For this review, take the finished solid that the model builds, in its own axes (mm). Face numbers are marked on the shaded views. A direction names the side the tool comes from. Round coordinates to 2 decimals unless told otherwise and drop trailing zeros. Loops run counter-clockwise (first coordinate to the right, second up) from the corner with the lowest first, then second, coordinate; pieces in that order, holes last.
1) Tool access review of the marked faces 4 and 5: name each direction out of +Z, -Z, +X, -X, +Y, -Y from which nothing blocks a thin tool from reaching the whole face with its end or side.
2) Take a section at B-B (x = 44.5). State the section outline as (y, z) points, then the cut area to 3 significant figures.
3) Insertion check: pin 1 (10 mm diameter, centred on y = -3, z = -6.5, fed in from -X); pin 2 (7.5 mm diameter, centred on x = 145, y = 5, fed in from +Z); pin 3 (6 mm diameter, centred on y = -7, z = -2.5, fed in from +X); pin 4 (5 mm diameter, centred on x = 139, y = 2, fed in from -Z). Each pin has a flat end and moves straight along its axis. Give the tip position at first contact, or say it passes through.
4) Mouldability with a two-part tool opening along X and no side actions: class the marked faces 1, 2 and 3 as pulls with the +X half, pulls with the -X half, needs draft (parallel to the pull), parting line crosses it, or undercut.
5) Take a section at A-A (x = 16). State the section outline as (y, z) points, then the cut area to 3 significant figures.
6) Wall thickness on L1, parallel to Z at x = 111, y = -9; L2, parallel to Y at x = 147, z = 1.5; L3, parallel to Z at x = 70.5, y = -5.75: over which ranges is each line inside the solid? List them lowest first.
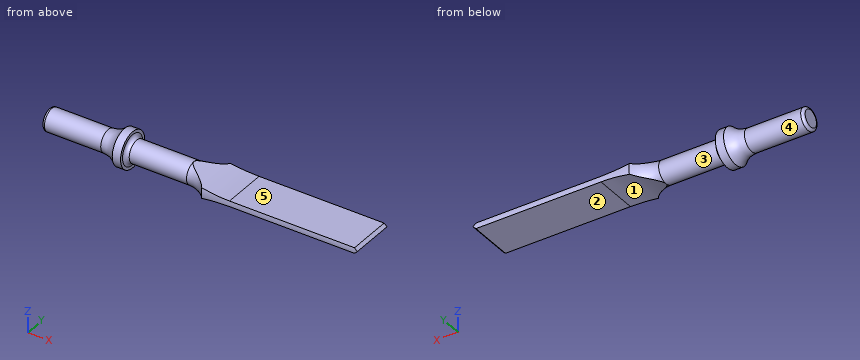
```python
from build123d import *

# Parameters (mm, degrees)
F3_DEPTH = 25.4
F4_DEPTH = 25.4
F6_DEPTH = 25.4
F7_DEPTH = 25.4


with BuildPart() as f1:
    # F0 (on Front) → F1 (revolve)
    with BuildSketch(Plane.XZ):
        with BuildLine():
            Line((0, 4.826), (0, 0))
            Line((0, 0), (184.15, 0))
            Line((184.15, 0), (184.15, 12.7))
            Line((184.15, 12.7), (95.25, 12.7))
            ThreePointArc((95.25, 12.7), (89.649516, 8.025968), (82.55, 6.35))
            Line((82.55, 6.35), (49.8856, 6.35))
            ThreePointArc((49.8856, 6.35), (48.269154, 7.019554), (47.5996, 8.636))
            Line((47.5996, 8.636), (47.5996, 10.3124))
            Line((47.5996, 10.3124), (42.8498, 10.3124))
            ThreePointArc((42.8498, 10.3124), (38.649372, 7.382577), (33.633274, 6.35))
            Line((33.633274, 6.35), (1.524, 6.35))
            ThreePointArc((1.524, 6.35), (0.446369, 5.903631), (0, 4.826))
        make_face()
    revolve(axis=Axis((92.075, 0, 0), (1, 0, 0)))

    # F2 (on Front) → F3 (cut)
    with BuildSketch(Plane.XZ):
        with BuildLine():
            Line((299.925119, 1.5875), (179.814342, 147.083428))
            ThreePointArc((179.814342, 147.083428), (30.837499, 128.380982), (111.256987, 1.5875))
            Line((111.256987, 1.5875), (299.925119, 1.5875))
        make_face()
        with BuildLine():
            Line((299.925119, -1.5875), (111.256987, -1.5875))
            ThreePointArc((111.256987, -1.5875), (30.837499, -128.380982), (179.814342, -147.083428))
            Line((179.814342, -147.083428), (299.925119, -1.5875))
        make_face()
    extrude(amount=-F3_DEPTH, mode=Mode.SUBTRACT)

    # F2 (on Front) → F4 (cut)
    with BuildSketch(Plane.XZ):
        with BuildLine():
            Line((299.925119, 1.5875), (179.814342, 147.083428))
            ThreePointArc((179.814342, 147.083428), (30.837499, 128.380982), (111.256987, 1.5875))
            Line((111.256987, 1.5875), (299.925119, 1.5875))
        make_face()
        with BuildLine():
            Line((299.925119, -1.5875), (111.256987, -1.5875))
            ThreePointArc((111.256987, -1.5875), (30.837499, -128.380982), (179.814342, -147.083428))
            Line((179.814342, -147.083428), (299.925119, -1.5875))
        make_face()
    extrude(amount=F4_DEPTH, mode=Mode.SUBTRACT)

    # F5 (on Front) → F6 (cut)
    with BuildSketch(Plane.XZ):
        Polygon((184.15, -3.802141), (184.15, 0), (180.61569, -3.53431), align=None)
        Polygon((180.61569, 3.53431), (184.15, 0), (184.15, 3.802141), align=None)
    extrude(amount=-F6_DEPTH, mode=Mode.SUBTRACT)

    # F5 (on Front) → F7 (cut)
    with BuildSketch(Plane.XZ):
        Polygon((180.61569, 3.53431), (184.15, 0), (184.15, 3.802141), align=None)
        Polygon((184.15, -3.802141), (184.15, 0), (180.61569, -3.53431), align=None)
    extrude(amount=F7_DEPTH, mode=Mode.SUBTRACT)


solid = f1.part
```
Response:
1. face 4: -X
1. face 5: +Z, +X, +Y, -Y
2. outline: circle Ø20.62 at (0, 0)
2. area: 334 mm2
3. pin 1: stops at x = 0
3. pin 2: stops at z = 1.59
3. pin 3: stops at x = 184.15
3. pin 4: stops at z = -1.59
4. face 1: pulls with the +X half
4. face 2: needs draft
4. face 3: undercut
5. outline: circle Ø12.7 at (0, 0)
5. area: 127 mm2
6. L1: z = -1.59 to 1.59
6. L2: y = -12.61 to 12.61
6. L3: z = -2.69 to 2.69
